Source: three-view drawing plus pictorial views. Frame: mm from the lowest corner of the part. A direction names the side the tool comes from. Give positions to 0.01 mm unless a question says otherwise; leave off trailing zeros. Order: outer loops, then holes, each group sorted by start corner. A loop starts at its lowest first (then second) coordinate and runs counter-clockwise, first axis right, second up. Notation, with made-up numbers: M 0,22 L 16,22 A18 cw 16,31 Z; hole C 62.25,74.5 d4. An arc over 180 degrees is marked long. Use CSV: the item, a comma, the result in double quotes. Start each with the question number.
1. Section query C-C, the plane x = 1. Return the cut outline in (y, z), plus the area to 3 significant figures.
2. Pin query (flat end, axial travel): P1, Ø2.5, axis at x = 6.25, y = 1.9, coming from the -Z side; P2, Ø4, axis at x = 4, y = 29.5, coming from the +Z side; P3, Ø3, axis at x = 2.5, z = 7, coming from the -Y side. Return the tip coordinate at first contact, or that it passes through.
3. Line query: line 1 along Y through (x, z) = (6.25, 18); line 2 along Y through (x, z) = (9.75, 7); line 3 along Z through (x, y) = (10, 29). Output: solid intervals per line, ascending. Write a range as [from, to].
4. Section query B-B, the plane x = 6.25. Return the cut outline in (y, z).
5. Reachability of the marked faces 1, 2, 3, 4 and 5 from +Z, -Z, +X, -X, +Y, -Y: full face, straight path, thin tool, end or side. Return the list, or none.
6. Section query D-D, the plane z = 12. Return the cut outline in (x, y), plus the area to 3 significant figures.
7. Section query A-A, the plane y = 1.9. Return the cut outline in (x, z).
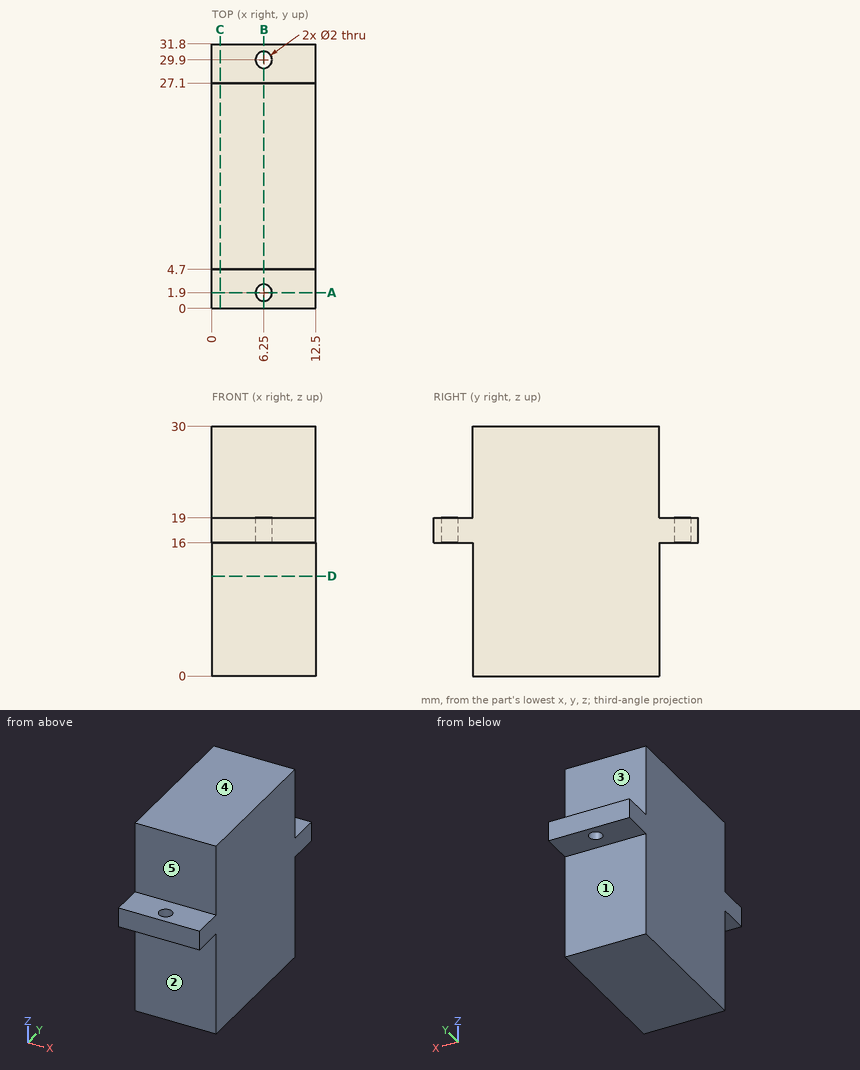
Result set:
1,outline,"M 0,16 L 4.7,16 L 4.7,0 L 27.1,0 L 27.1,16 L 31.8,16 L 31.8,19 L 27.1,19 L 27.1,30 L 4.7,30 L 4.7,19 L 0,19 Z"
1,area,"700 mm2"
2,P1,"z = 16"
2,P2,"z = 19"
2,P3,"y = 4.7"
3,line 1,"[0, 0.9], [2.9, 28.9], [30.9, 31.8]"
3,line 2,"[4.7, 27.1]"
3,line 3,"[16, 19]"
4,outline,"M 0,16 L 0.9,16 L 0.9,19 L 0,19 Z; M 2.9,16 L 4.7,16 L 4.7,0 L 27.1,0 L 27.1,16 L 28.9,16 L 28.9,19 L 27.1,19 L 27.1,30 L 4.7,30 L 4.7,19 L 2.9,19 Z; M 30.9,16 L 31.8,16 L 31.8,19 L 30.9,19 Z"
5,face 1,"-Z, +X, -X, +Y"
5,face 2,"-Z, +X, -X, -Y"
5,face 3,"+Z, +X, -X, +Y"
5,face 4,"+Z, +X, -X, +Y, -Y"
5,face 5,"+Z, +X, -X, -Y"
6,outline,"M 0,4.7 L 12.5,4.7 L 12.5,27.1 L 0,27.1 Z"
6,area,"280 mm2"
7,outline,"M 0,16 L 5.25,16 L 5.25,19 L 0,19 Z; M 7.25,16 L 12.5,16 L 12.5,19 L 7.25,19 Z"
